Geometry: see drawing. Coordinates: mm, zero at the bounding-box minimum. A direction names the side the tool comes from. Coordinates: 2 decimals unless noted, no trailing zeros. Loops run counter-clockwise (first coordinate to the right, second up) from the corner with the lowest first, then second, coordinate; pieces in that order, holes last. Notation, with made-up numbers: (-21, 31.5) - (-11, 31.5) arc R31 cw to (-11, 60.5) - close; hole circle Ø11 at (50.5, -2). An arc over 180 degrees is marked (long way). Use a Markdown table: item, result. Add a question column.
1. Access query for the marked faces 1 and 2. Directions: +Z, -Z, +X, -X, +Y, -Y. A direction counts if a zero-diameter tool reaches every point of the face in a straight line with its end or side. Return the directions, or none.
2. Contact query for flat-ended pins moving along their axis: P1, Ø6, axis at x = 22.5, z = 16, coming from the +Y side (3 decimals); P2, Ø8, axis at y = 20.5, z = 21.5, coming from the +X side (3 decimals). Output: stop coordinate, or through.
3. Section query D-D on z = 5.5. Return the cut outline in (x, y) (1 decimal), then the cut area to 3 significant figures.
4. Ray query, L1, parallel to X at y = 1.5, z = 12.7; L2, parallel to Z at x = 38, y = 1; L3, parallel to Y at x = 30.5, z = 15.75 (1 decimal). Return the intervals inside material, ascending. Write a range as [from, to].
5. Section query B-B on z = 12.7. Return the cut outline in (x, y) (1 decimal).
6. Section query C-C on x = 12.7. Return the cut outline in (y, z) (1 decimal).
7. Section query A-A on y = 38.1. Return the cut outline in (x, z) (1 decimal).
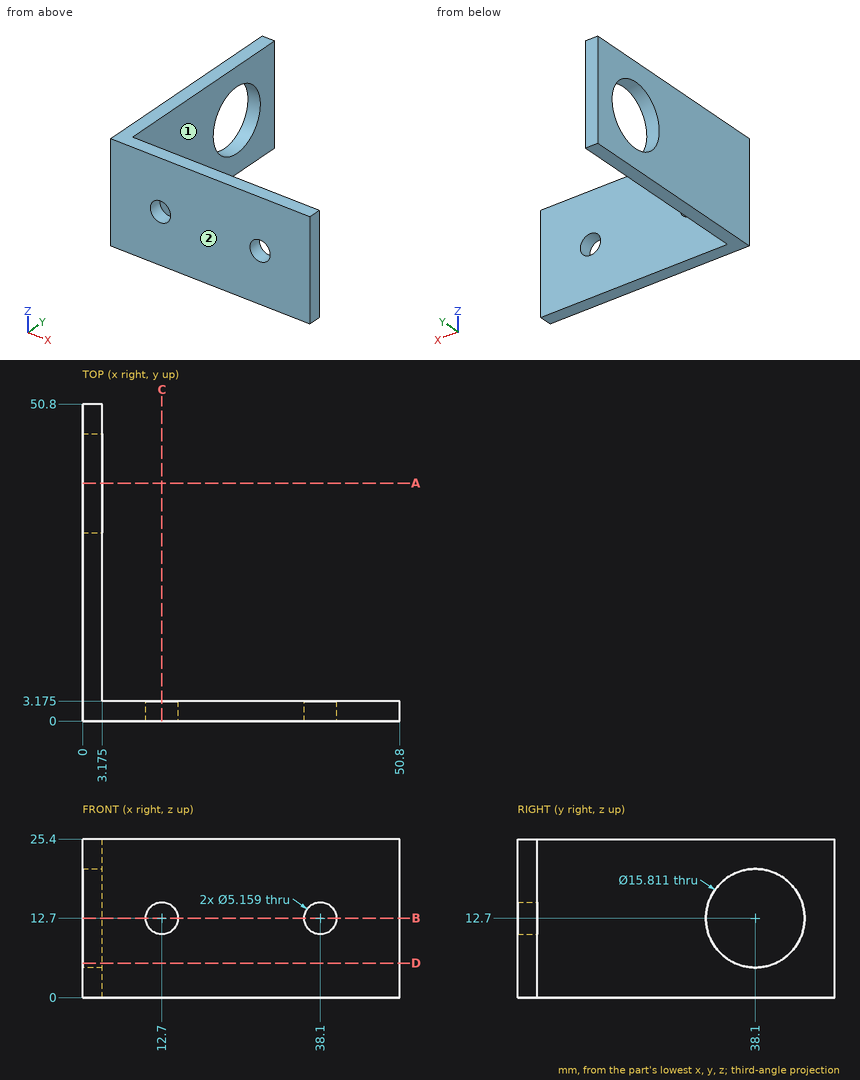
Resolved:
| question | item | result |
|---|---|---|
| 1 | face 1 | +Z, -Z, +X, +Y |
| 1 | face 2 | +Z, -Z, +X, -X, -Y |
| 2 | P1 | y = 3.175 |
| 2 | P2 | x = 3.175 |
| 3 | outline | (0, 0) - (50.8, 0) - (50.8, 3.2) - (3.2, 3.2) - (3.2, 34.8) - (0, 34.8) - close; (0, 41.4) - (3.2, 41.4) - (3.2, 50.8) - (0, 50.8) - close |
| 3 | area | 292 mm² |
| 4 | L1 | [0, 10.12], [15.28, 35.52], [40.68, 50.8] |
| 4 | L2 | [0, 10.12], [15.28, 25.4] |
| 4 | L3 | [0, 3.2] |
| 5 | outline | (0, 0) - (10.1, 0) - (10.1, 3.2) - (3.2, 3.2) - (3.2, 30.2) - (0, 30.2) - close; (0, 46) - (3.2, 46) - (3.2, 50.8) - (0, 50.8) - close; (15.3, 0) - (35.5, 0) - (35.5, 3.2) - (15.3, 3.2) - close; (40.7, 0) - (50.8, 0) - (50.8, 3.2) - (40.7, 3.2) - close |
| 6 | outline | (0, 0) - (3.2, 0) - (3.2, 10.1) - (0, 10.1) - close; (0, 15.3) - (3.2, 15.3) - (3.2, 25.4) - (0, 25.4) - close |
| 7 | outline | (0, 0) - (3.2, 0) - (3.2, 4.8) - (0, 4.8) - close; (0, 20.6) - (3.2, 20.6) - (3.2, 25.4) - (0, 25.4) - close |
